from build123d import *

# Parameters (mm, degrees)
F0_W     = 2000
F0_H     = 500
F1_DEPTH = 1000
F2_W     = 1797.439754
F2_H     = 308.463849
F3_DEPTH = 1000.001
F4_R     = 50
F5_W     = 773.947201
F5_H     = 195.373047
F6_DEPTH = 2000.001
F7_R     = 50


with BuildPart() as f1:
    # F0 (on Front) → F1 (new body)
    with BuildSketch(Plane.XZ):
        with Locations((0, -36.538462)):
            Rectangle(F0_W, F0_H)
    extrude(amount=F1_DEPTH)

    # F2 (on face) → F3 (cut, through all)
    with BuildSketch(Plane.XZ.offset(1000)):
        with Locations((1.209587, -38.093578)):
            Rectangle(F2_W, F2_H)
    extrude(amount=-F3_DEPTH, mode=Mode.SUBTRACT)

    # F4
    f4_edges = [f1.edges().sort_by_distance(p)[0] for p in [
        (1000, -500, 213.461538),
        (1000, -500, -286.538462),
        (-1000, -500, 213.461538),
        (-1000, -500, -286.538462),
        (-897.51029, -500, 116.138346),
        (-897.51029, -500, -192.325503),
        (899.929464, -500, 116.138346),
        (899.929464, -500, -192.325503),
    ]]
    fillet(f4_edges, radius=F4_R)

    # F5 (on face) → F6 (cut, through all)
    with BuildSketch(Plane(origin=(-1000, 0, 0), x_dir=(0, -1, 0), z_dir=(-1, 0, 0))):
        with Locations((502.068478, -36.354279)):
            Rectangle(F5_W, F5_H)
    extrude(amount=-F6_DEPTH, mode=Mode.SUBTRACT)

    # F7
    f7_edges = [f1.edges().sort_by_distance(p)[0] for p in [
        (949.964732, -115.094878, 61.332244),
        (-948.755145, -115.094878, 61.332244),
        (949.964732, -889.042079, 61.332244),
        (-948.755145, -889.042079, 61.332244),
        (949.964732, -115.094878, -134.040803),
        (-948.755145, -115.094878, -134.040803),
        (949.964732, -889.042079, -134.040803),
        (-948.755145, -889.042079, -134.040803),
    ]]
    fillet(f7_edges, radius=F7_R)


solid = f1.part
Geometry check sheet. Reference: the model listing, model coordinates, mm. A direction names the side the tool comes from. Round coordinates to 2 decimals unless told otherwise and drop trailing zeros. Order: outer loops, then holes, each group sorted by start corner. A loop starts at its lowest first (then second) coordinate and runs counter-clockwise, first axis right, second up. Notation, with made-up numbers: M 32.5,43 L 53.5,43 A20 ccw 53.5,78 Z; hole C -13.5,29 d8. An arc over 180 degrees is marked long. Write each question's results on one line, items separated by ' | '. Start each with the question number.
1. Set-up check for faces 1 (the face through (-882.475, -493, 101.88)), 2 (the face through (950.67, -874.01, -119.78)), 3 (the face through (-13, -493, 213.462)): record each of +Z, -Z, +X, -X, +Y, -Y from which the full face is reachable in a straight line by a thin tool's end or side.
2. Cross-section at C-C on z = -46. Record the boundary of the cut face in (x, y), plus the area to 3 significant figures.
3. Draft check along Y on faces 4 (the face through (-949, -889.042, -37)), 5 (the face through (-897.51, -428, -139)), 6 (the face through (-14, -1000, 134)). Enter one of: pulls with the +Y half, pulls with the -Y half, needs draft (parallel to the pull), parting line crosses it, or undercut.
4. Material ranges on L1, parallel to Z at x = 247, y = -666; L2, parallel to Z at x = 918, y = -339.5; L3, parallel to X at y = -80.5, z = -99, recorded low to high. Write a range as from..to.
5. Cross-section at D-D on x = 876. Record the boundary of the cut face in (y, z).
6. Cross-section at B-B on y = -634.5. Record the boundary of the cut face in (x, z).
7. Go/stop test with a flat-tipped pin: P1, Ø1.5, axis at x = 195, z = -235, coming from the +Y side. Record where the tip stops, or that it passes through.
8. Cross-section at A-A on x = -72. Record the boundary of the cut face in (y, z), plus the area to 3 significant figures.
Resolved:
1) face 1: +Y, -Y | face 2: +X, -X | face 3: +Z, +X, -X, +Y, -Y
2) outline: M -1000,-1000 L -897.51,-1000 L -897.51,-889.04 L -1000,-889.04 Z; M -1000,-115.09 L -897.51,-115.09 L -897.51,0 L -1000,0 Z; M 899.93,-1000 L 1000,-1000 L 1000,-889.04 L 899.93,-889.04 Z; M 899.93,-115.09 L 1000,-115.09 L 1000,0 L 899.93,0 Z | area: 45,800 mm2
3) face 4: undercut | face 5: needs draft | face 6: pulls with the -Y half
4) L1: -286.54..-192.33, 116.14..213.46 | L2: -286.54..-134.04, 61.33..213.46 | L3: -1000..-897.51, 899.93..1000
5) outline: M -1000,-286.54 L 0,-286.54 L 0,-184.99 L -1000,-184.99 Z; M -1000,108.8 L 0,108.8 L 0,213.46 L -1000,213.46 Z
6) outline: M -1000,-236.54 A50 ccw -950,-286.54 L 950,-286.54 A50 ccw 1000,-236.54 L 1000,-134.04 L 899.93,-134.04 L 899.93,-142.33 A50 cw 849.93,-192.33 L -847.51,-192.33 A50 cw -897.51,-142.33 L -897.51,-134.04 L -1000,-134.04 Z; M -1000,61.33 L -897.51,61.33 L -897.51,66.14 A50 cw -847.51,116.14 L 849.93,116.14 A50 cw 899.93,66.14 L 899.93,61.33 L 1000,61.33 L 1000,163.46 A50 ccw 950,213.46 L -950,213.46 A50 ccw -1000,163.46 Z
7) P1: y = 0
8) outline: M -1000,-286.54 L 0,-286.54 L 0,-192.33 L -1000,-192.33 Z; M -1000,116.14 L 0,116.14 L 0,213.46 L -1000,213.46 Z | area: 192,000 mm2
